```python
from build123d import *

# Parameters (mm, degrees)
BOSS_EXTRUDE1_DEPTH = 3.175
SKETCH2_W           = 6.604
SKETCH2_H           = 12.7
SKETCH2_W_2         = 50.8
SKETCH2_H_2         = 4.7625
CUT_EXTRUDE1_DEPTH  = 192.297317003


with BuildPart() as part:
    # Sketch1 → Boss-Extrude1 (new body)
    with BuildSketch(Plane.XY):
        Polygon((95.25, 0), (-95.25, 0), (-153.67, -101.186408178), (-131.672954744, -113.886408178), (-80.585303163, -25.4), (80.585303163, -25.4), (131.672954744, -113.886408178), (153.67, -101.186408178), align=None)
    extrude(amount=BOSS_EXTRUDE1_DEPTH)

    # Sketch2 → Cut-Extrude1 (cut, through all)
    with BuildSketch(Plane.XY.offset(3.175)):
        with Locations((0, -6.35)):
            Rectangle(SKETCH2_W, SKETCH2_H)
        Polygon((-111.506, -28.156217928), (-136.906, -72.15030844), (-132.781554014, -74.53155844), (-107.381554014, -30.537467928), align=None)
        with Locations((-50.8, -2.38125)):
            Rectangle(SKETCH2_W_2, SKETCH2_H_2)
        with Locations((50.8, -2.38125)):
            Rectangle(SKETCH2_W_2, SKETCH2_H_2)
        Polygon((107.381554014, -30.537467928), (111.506, -28.156217928), (136.906, -72.15030844), (132.781554014, -74.53155844), align=None)
        Polygon((-152.4, -98.986703653), (-123.070606325, -98.986703653), (-131.672954744, -113.886408178), (-153.67, -101.186408178), align=None)
        Polygon((153.67, -101.186408178), (152.4, -98.986703653), (123.070606325, -98.986703653), (131.672954744, -113.886408178), align=None)
    extrude(amount=-CUT_EXTRUDE1_DEPTH, mode=Mode.SUBTRACT)


solid = part.part
```
Work out the finished part from the listing and answer in its coordinate system (mm). Give positions to 0.01 mm unless a question says otherwise; leave off trailing zeros. Write each loop counter-clockwise with the first axis right and the second up, starting at its lowest first coordinate (ties: lowest second). Pieces come first, ordered by that corner, then holes. Notation, with made-up numbers: (-22, -35) - (34, -35) arc R7 ccw to (34, -29) - close; hole circle Ø8 at (33.25, 83). An arc over 180 degrees is marked (long way). Use one line per item in the form item = value.
1. A cutting plane is placed at B-B (y = -37). Write down the section's boundary in (x, z) (3 decimals).
Filled in:
outline = (-111.113, 0) - (-87.283, 0) - (-87.283, 3.175) - (-111.113, 3.175) - close; (87.283, 0) - (111.113, 0) - (111.113, 3.175) - (87.283, 3.175) - close
2. Determine the mould class of faces 1 (the face through (-144.545, -85.381, 1.565)), 2 (the face through (-102.125, -62.708, 1.565)), 3 (the face through (101.53, -61.68, 1.57)), 4 (the face through (-1, -16, 3.175)) for opening direction X: released by +X, released by -X, zero draft, split by the parting line, or undercut.
Filled in:
face_1 = released by -X
face_2 = undercut
face_3 = undercut
face_4 = zero draft
3. Each of these flat-tipped pins is pushed along its axis until it touches: pin 1 Ø1 at (y, z) = (-6, 2) entering from +X; pin 2 Ø1.5 at (x, z) = (38.5, 1.5) entering from +Y; pin 3 Ø1.6 at (y, z) = (-2.5, 1) entering from +X. Where does it stop, or does it pass through?
Filled in:
pin_1 = 99
pin_2 = -4.76
pin_3 = 97.16
4. A cutting plane is placed at C-C (x = 68). Write down the section's boundary in (y, z) (1 decimal).
Filled in:
outline = (-25.4, 0) - (-4.8, 0) - (-4.8, 3.2) - (-25.4, 3.2) - close
5. Consider L1, parallel to Y at x = 71, z = 0.85; L2, parallel to X at y = -8.5, z = 0.65; L3, parallel to X at y = -9, z = 3. Determine where each line is inside the solid, lowest interval first.
Filled in:
L1 = -25.4 to -4.76
L2 = -100.16 to -3.3, 3.3 to 100.16
L3 = -100.45 to -3.3, 3.3 to 100.45
6. A cutting plane is placed at A-A (z = 2). Write down the section's boundary in (x, y), and give its area (3 significant figures).
Filled in:
outline = (-152.4, -98.99) - (-123.07, -98.99) - (-80.59, -25.4) - (80.59, -25.4) - (123.07, -98.99) - (152.4, -98.99) - (136.91, -72.15) - (132.78, -74.53) - (107.38, -30.54) - (111.51, -28.16) - (95.25, 0) - (76.2, 0) - (76.2, -4.76) - (25.4, -4.76) - (25.4, 0) - (3.3, 0) - (3.3, -12.7) - (-3.3, -12.7) - (-3.3, 0) - (-25.4, 0) - (-25.4, -4.76) - (-76.2, -4.76) - (-76.2, 0) - (-95.25, 0) - (-111.51, -28.16) - (-107.38, -30.54) - (-132.78, -74.53) - (-136.91, -72.15) - close
area = 8,480 mm^2
